```python
from build123d import *

# Parameters (mm, degrees)
SKETCH1_R           = 14
BOSS_EXTRUDE1_DEPTH = 26
SKETCH2_R           = 4
BOSS_EXTRUDE2_DEPTH = 7
SKETCH3_R           = 3
BOSS_EXTRUDE3_DEPTH = 7
SKETCH5_R           = 5
CUT_EXTRUDE1_DEPTH  = 5
SKETCH7_R           = 7
CUT_EXTRUDE2_DEPTH  = 5
FILLET1_R           = 2
SKETCH9_RX          = 7.5
SKETCH9_RY          = 4.068391424
SKETCH9_RY_2        = 3.899393896
CUT_EXTRUDE3_DEPTH  = 4
SKETCH11_R          = 14
SKETCH11_R_2        = 8
CUT_EXTRUDE4_DEPTH  = 1


with BuildPart() as part:
    # Sketch1 → Boss-Extrude1 (new body)
    with BuildSketch(Plane(origin=(0, 0, 0), x_dir=(1, 0, 0), z_dir=(0, 1, 0))):
        with Locations(Location((0, 0, 0), (0, 0, 90))):
            Circle(SKETCH1_R)
    extrude(amount=BOSS_EXTRUDE1_DEPTH)

    # Sketch2 → Boss-Extrude2 (add)
    with BuildSketch(Plane(origin=(0, 26, 0), x_dir=(1, 0, 0), z_dir=(0, 1, 0))):
        with Locations(Location((0, 0, 0), (0, 0, 270))):
            Circle(SKETCH2_R)
    extrude(amount=BOSS_EXTRUDE2_DEPTH)

    # Sketch3 → Boss-Extrude3 (add)
    with BuildSketch(Plane(origin=(0, 33, 0), x_dir=(1, 0, 0), z_dir=(0, 1, 0))):
        with Locations(Location((0, 0, 0), (0, 0, 270))):
            Circle(SKETCH3_R)
    extrude(amount=BOSS_EXTRUDE3_DEPTH)

    # Sketch5 → Cut-Extrude1 (cut)
    with BuildSketch(Plane.XZ):
        with Locations(Location((0, 0, 0), (0, 0, 270))):
            Circle(SKETCH5_R)
    extrude(amount=-CUT_EXTRUDE1_DEPTH, mode=Mode.SUBTRACT)

    # Sketch7 → Cut-Extrude2 (cut)
    with BuildSketch(Plane(origin=(0, 26, 0), x_dir=(1, 0, 0), z_dir=(0, 1, 0))):
        with Locations((-13.099617669, 4.939637327)):
            Circle(SKETCH7_R)
        with Locations((-8.745866262, -10.932054854)):
            Circle(SKETCH7_R)
        with Locations((7.694394058, -11.695995045)):
            Circle(SKETCH7_R)
        with Locations((13.501246597, 3.703557793)):
            Circle(SKETCH7_R)
        with Locations((0.649805899, 13.984911594)):
            Circle(SKETCH7_R)
    extrude(amount=-CUT_EXTRUDE2_DEPTH, mode=Mode.SUBTRACT)

    # Fillet1
    fillet1_edges = [part.edges().sort_by_distance(p)[0] for p in [
        (-13.501257172, 26, 3.703519243),
        (-0.64984583, 26, 13.984909739),
        (13.099631773, 26, 4.939599924),
        (8.745835048, 26, -10.932079826),
        (-7.694394058, 26, -11.695995045),
    ]]
    fillet(fillet1_edges, radius=FILLET1_R)

    # Sketch9 → Cut-Extrude3 (cut)
    with BuildSketch(Plane.XZ):
        with Locations(Location((0, -14), (0, 0, -90))):
            Ellipse(SKETCH9_RX, SKETCH9_RY)
        with Locations(Location((14, 0), (0, 0, 0))):
            Ellipse(SKETCH9_RX, SKETCH9_RY_2)
        with Locations(Location((0, 14), (0, 0, 90))):
            Ellipse(SKETCH9_RX, SKETCH9_RY)
        with BuildLine():
            ThreePointArc((-12.493901532, 6.31683659), (-14, 0), (-12.493901532, -6.31683659))
            add(Edge.make_bspline(
                [(-12.493901532, -6.31683659), (-7.506098468, 0), (-12.493901532, 6.31683659)],
                knots=[0, 0, 0, 1, 1, 1], degree=2))
        make_face()
    extrude(amount=-CUT_EXTRUDE3_DEPTH, mode=Mode.SUBTRACT)

    # Sketch11 → Cut-Extrude4 (cut)
    with BuildSketch(Plane(origin=(0, 5, 0), x_dir=(-1, 0, 0), z_dir=(0, -1, 0))):
        with Locations(Location((0, 0, 0), (0, 0, 90))):
            Circle(SKETCH11_R)
        with Locations(Location((0, 0, 0), (0, 0, 90))):
            Circle(SKETCH11_R_2, mode=Mode.SUBTRACT)
    extrude(amount=-CUT_EXTRUDE4_DEPTH, mode=Mode.SUBTRACT)


solid = part.part
```
Model file for the job. Use its own axes, mm. A direction names the side the tool comes from. Give positions to 0.01 mm unless a question says otherwise; leave off trailing zeros. Loops run counter-clockwise (first coordinate to the right, second up) from the corner with the lowest first, then second, coordinate; pieces in that order, holes last. Notation, with made-up numbers: (36, 32) - (87, 32) arc R24 cw to (87, 66) - close; hole circle Ø2 at (83, 13.25). An arc over 180 degrees is marked (long way). One line per item, written item: value. Start each with the question number.
1. Slice it at B-B (y = 30). List the corners of the cut face in (x, z), plus the area to 3 significant figures.
2. Pin check, flat tips, straight feed: pin 1 (6 mm diameter, centred on y = 11, z = 4, fed in from +X); pin 2 (6 mm diameter, centred on y = 26.5, z = 0, fed in from -X); pin 3 (2 mm diameter, centred on x = -8, z = -9, fed in from +Y). Stop position of each tip, or through.
3. Probe L1, parallel to X at y = 2.55, z = 0; L2, parallel to Y at x = 7, z = -0.5; L3, parallel to Y at x = 12.25, z = -1. List the from-to ranges inside material, lowest first. Write a range as from..to.
4. Which spindle directions (+Z, -Z, +X, -X, +Y, -Y) get a long thin tool onto all of the face, cutting with end or side? Do faces 1 (the flat face through (0, 4, -11)), 2 (the flat face through (0, 21, -11)), 3 (the cylindrical face through (-4.27, 23.54, 5.55)). Say none if no direction does.
5. Slice it at A-A (y = 11.5). List the corners of the cut face in (x, z), plus the area to 3 significant figures.
6. Pull direction Y, two halves, no side cores. Call faces 4 (the cylindrical face through (-7.81, 5.49, 1.73)), 5 (the flat face through (11, 4, 0)), 6 (the flat face through (6, 21, 9)): pulls with the +Y half, pulls with the -Y half, needs draft (parallel to the pull), parting line crosses it, or undercut.
Solution:
1. outline: circle Ø8 at (0, 0)
1. area: 50.3 mm^2
2. pin 1: stops at x = 13.96
2. pin 2: stops at x = -13.83
2. pin 3: stops at y = 26
3. L1: x = -10..-5, 5..6.5
3. L2: y = 4..26
3. L3: y = 4..5, 6..21
4. face 1: -Z, -Y
4. face 2: -Z, +Y
4. face 3: +Y
5. outline: circle Ø28 at (0, 0)
5. area: 616 mm^2
6. face 4: undercut
6. face 5: pulls with the -Y half
6. face 6: pulls with the +Y half
